from build123d import *

# Parameters (mm, degrees)
SKETCH1_R           = 1
BOSS_EXTRUDE1_DEPTH = 0.8
BOSS_EXTRUDE4_DEPTH = 5


with BuildPart() as part:
    # Sketch1 → Boss-Extrude1 (new body)
    with BuildSketch(Plane(origin=(0, 0, 0), x_dir=(1, 0, 0), z_dir=(0, 1, 0))):
        with BuildLine():
            Line((6.5, 1.5), (0.738689027, 2.388375708))
            ThreePointArc((0.738689027, 2.388375708), (-2.5, 0), (0.738689027, -2.388375708))
            Line((0.738689027, -2.388375708), (6.5, -1.5))
            Line((6.5, -1.5), (10, -1.5))
            Line((10, -1.5), (10, 1.5))
            Line((10, 1.5), (6.5, 1.5))
        make_face()
        with Locations(Location((0, 0, 0), (0, 0, 270))):
            Circle(SKETCH1_R, mode=Mode.SUBTRACT)
    extrude(amount=BOSS_EXTRUDE1_DEPTH)

    # Sketch5 → Boss-Extrude4 (add)
    with BuildSketch(Plane(origin=(10, 0, 0), x_dir=(0, 0, -1), z_dir=(1, 0, 0))):
        with BuildLine():
            ThreePointArc((1.356465997, 0.8), (1.500836816, 1.162716057), (1.55, 1.55))
            ThreePointArc((1.55, 1.55), (-0.387283943, 3.050836816), (-1.356465997, 0.8))
            Line((-1.356465997, 0.8), (-0.9367497, 0.8))
            ThreePointArc((-0.9367497, 0.8), (-0.397429466, 2.682276388), (1.2, 1.55))
            ThreePointArc((1.2, 1.55), (1.132276388, 1.152570534), (0.9367497, 0.8))
            Line((0.9367497, 0.8), (1.356465997, 0.8))
        make_face()
        with BuildLine():
            Line((-0.9367497, 0.8), (-1.356465997, 0.8))
            ThreePointArc((-1.356465997, 0.8), (0, 0), (1.356465997, 0.8))
            Line((1.356465997, 0.8), (0.9367497, 0.8))
            ThreePointArc((0.9367497, 0.8), (0, 0.35), (-0.9367497, 0.8))
        make_face()
    extrude(amount=-BOSS_EXTRUDE4_DEPTH)


solid = part.part
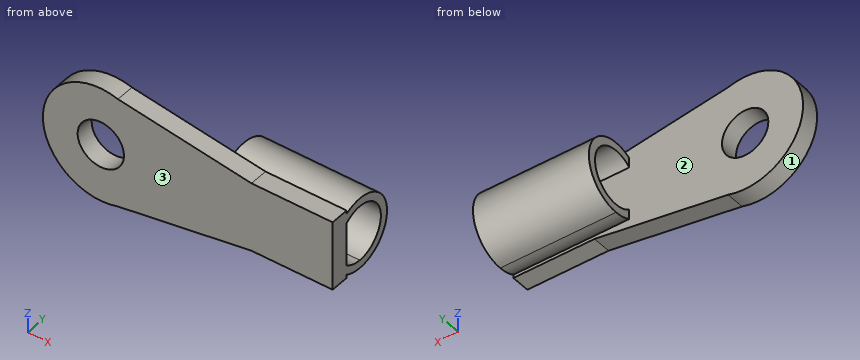
The model under review builds one solid part; all positions refer to its coordinate system, in mm. Face numbers are marked on the shaded views. Round coordinates to 2 decimals unless told otherwise and drop trailing zeros. Loops run counter-clockwise (first coordinate to the right, second up) from the corner with the lowest first, then second, coordinate; pieces in that order, holes last. Notation, with made-up numbers: (28.5, 1.5) -> (42.5, 1.5) arc R22 cw to (42.5, 12.5) -> close; hole circle Ø9 at (-32.5, 19). An arc over 180 degrees is marked (long way). Return JSON: item names as keys, results as strings.
(1) Add section D-D on x = 7.5. Write out the cut boundary in (y, z), plus the area to 3 significant figures.
Solved:
{"outline": "(0, -1.5) -> (0.8, -1.5) -> (0.8, -1.36) arc R1.55 ccw (long way) to (0.8, 1.36) -> (0.8, 1.5) -> (0, 1.5) -> close; hole (0.8, -0.94) arc R1.2 ccw (long way) to (0.8, 0.94) -> close", "area": "4.47 mm2"}
(2) The part is to be moulded in two halves that separate along Y. For the marked faces 1, 2 and 3, say which applies: released by +Y, released by -Y, zero draft, split by the parting line, or undercut.
Solved:
{"face 1": "zero draft", "face 2": "undercut", "face 3": "released by -Y"}
(3) Add section B-B on x = 0. Write out the cut boundary in (y, z), plus the area to 3 significant figures.
Solved:
{"outline": "(0, -2.5) -> (0.8, -2.5) -> (0.8, -1) -> (0, -1) -> close; (0, 1) -> (0.8, 1) -> (0.8, 2.5) -> (0, 2.5) -> close", "area": "2.40 mm2"}
(4) For line 1 (Y direction, x = 3.5, z = -0.75); line 2 (Y direction, x = 5.75, z = 0.1); line 3 (X direction, y = 0.6, z = 0.3), list the stretches that pass through material, from the lowest coordinate up.
Solved:
{"line 1": "0 to 0.8", "line 2": "0 to 0.8, 2.75 to 3.1", "line 3": "-2.48 to -0.95, 0.95 to 10"}
(5) Add section A-A on z = 0. Write out the cut boundary in (x, y).
Solved:
{"outline": "(-2.5, 0) -> (-1, 0) -> (-1, 0.8) -> (-2.5, 0.8) -> close; (1, 0) -> (10, 0) -> (10, 0.8) -> (1, 0.8) -> close; (5, 2.75) -> (10, 2.75) -> (10, 3.1) -> (5, 3.1) -> close"}
(6) For pin 1 (0.6 mm diameter, centred on x = 8.5, y = 0.5, fed in from +Z); pin 2 (1.5 mm diameter, centred on x = 3.5, z = -1, fed in from +Y); pin 3 (0.9 mm diameter, centred on x = 8.5, y = 0.5, fed in from -Z), all flat-tipped, find the tip position at first contact; note any pin that passes through.
Solved:
{"pin 1": "z = 1.5", "pin 2": "y = 0.8", "pin 3": "z = -1.5"}
(7) Add section C-C on y = 2.55. Write out the cut boundary in (x, z).
Solved:
{"outline": "(5, -1.18) -> (10, -1.18) -> (10, -0.66) -> (5, -0.66) -> close; (5, 0.66) -> (10, 0.66) -> (10, 1.18) -> (5, 1.18) -> close"}
